Check sheet for the drawn part. Datum: minimum x, y, z corner. Units: mm. Round coordinates to 2 decimals unless told otherwise and drop trailing zeros. Write each loop counter-clockwise with the first axis right and the second up, starting at its lowest first coordinate (ties: lowest second). Pieces come first, ordered by that corner, then holes. Notation, with made-up numbers: (-22, 15.25) - (-17, 15.25) arc R27 ccw to (-17, 44.25) - close; hole circle Ø3 at (22, -32.75). An arc over 180 degrees is marked (long way). Answer as a JSON object with one key per item and string values.
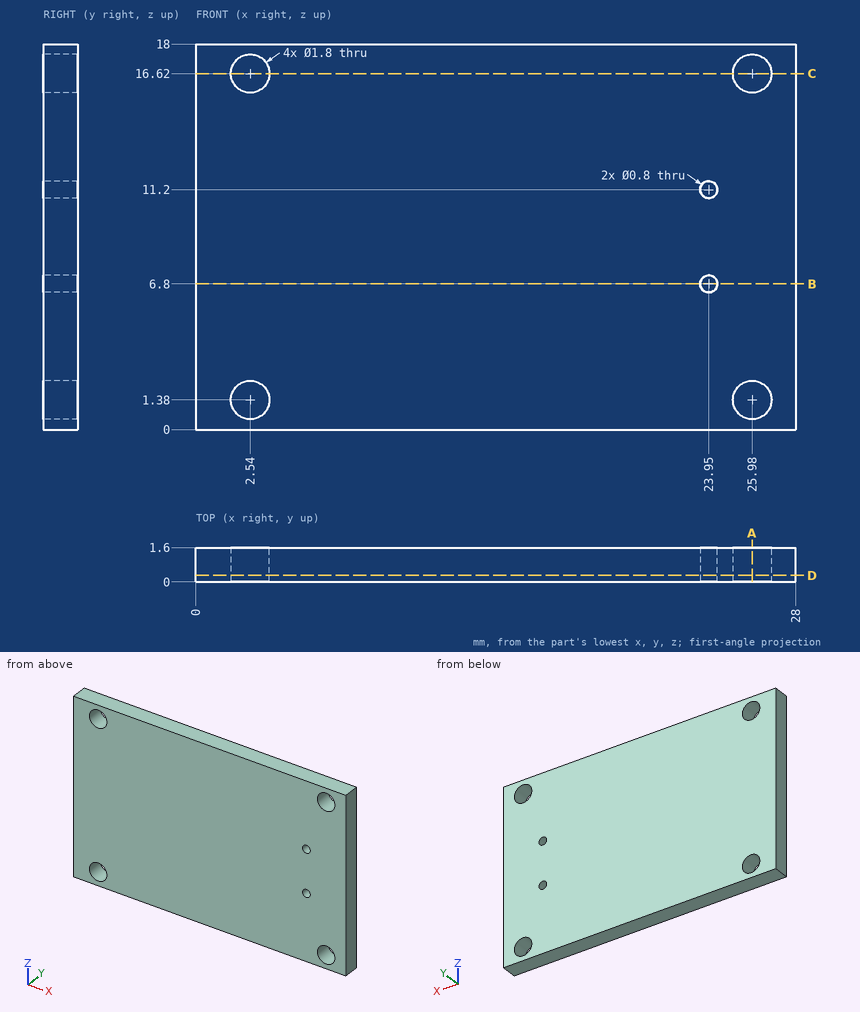
Q1. Material ranges on line 1 along Z through (x, y) = (2.54, 1.1); line 2 along X through (y, z) = (0.5, 16.62); line 3 along Z through (x, y) = (23.95, 0.7), recorded low to high. Write a range as [from, to].
Geometry check:
{"line 1": "z = [0, 0.48], [2.28, 15.72], [17.52, 18]", "line 2": "x = [0, 1.64], [3.44, 25.08], [26.88, 28]", "line 3": "z = [0, 6.4], [7.2, 10.8], [11.6, 18]"}
Q2. Section check A-A, the plane x = 25.98. Record the cut outline in (y, z).
Geometry check:
{"outline": "(0, 0) - (1.6, 0) - (1.6, 0.48) - (0, 0.48) - close; (0, 2.28) - (1.6, 2.28) - (1.6, 15.72) - (0, 15.72) - close; (0, 17.52) - (1.6, 17.52) - (1.6, 18) - (0, 18) - close"}
Q3. Gauge pin test, flat end, axial feed: P1, Ø2.5, axis at x = 2.54, z = 16.62, coming from the -Y side. Record the tip position at first contact, or that the pin passes through.
Geometry check:
{"P1": "stops at y = 0"}
Q4. Section check B-B, the plane z = 6.8. Record the cut outline in (x, y).
Geometry check:
{"outline": "(0, 0) - (23.55, 0) - (23.55, 1.6) - (0, 1.6) - close; (24.35, 0) - (28, 0) - (28, 1.6) - (24.35, 1.6) - close"}
Q5. Section check D-D, the plane y = 0.3. Record the cut outline in (x, z).
Geometry check:
{"outline": "(0, 0) - (28, 0) - (28, 18) - (0, 18) - close; hole circle Ø1.8 at (2.54, 1.38); hole circle Ø1.8 at (2.54, 16.62); hole circle Ø0.8 at (23.95, 6.8); hole circle Ø0.8 at (23.95, 11.2); hole circle Ø1.8 at (25.98, 1.38); hole circle Ø1.8 at (25.98, 16.62)"}
Q6. Section check C-C, the plane z = 16.62. Record the cut outline in (x, y), then the cut area to 3 significant figures.
Geometry check:
{"outline": "(0, 0) - (1.64, 0) - (1.64, 1.6) - (0, 1.6) - close; (3.44, 0) - (25.08, 0) - (25.08, 1.6) - (3.44, 1.6) - close; (26.88, 0) - (28, 0) - (28, 1.6) - (26.88, 1.6) - close", "area": "39.0 mm2"}
